Read the model definition and answer for the solid it produces. Units are mm, in the model's axes. A direction names the side the tool comes from. Coordinates: 2 decimals unless noted, no trailing zeros. Loops run counter-clockwise (first coordinate to the right, second up) from the corner with the lowest first, then second, coordinate; pieces in that order, holes last. Notation, with made-up numbers: M 26,62.5 L 39,62.5 A19 cw 39,97.5 Z; hole C 18.25,44.5 d10. An arc over 180 degrees is marked long. Put each result on its own line as item: value.
from build123d import *

# Parameters (mm, degrees)
F1_DEPTH = 38.1
F5_DEPTH = 38.1
F6_DEPTH = 38.1
F7_W     = 25.4
F7_H     = 7.62
F8_DEPTH = 38.1


with BuildPart() as f1:
    # F0 (on Front) → F1 (new body)
    with BuildSketch(Plane.XZ):
        Polygon((6.35, 38.1), (0, 0), (6.35, 0), (11.43, 22.225), (16.51, 9.525), (21.59, 9.525), (26.67, 22.225), (31.75, 0), (38.1, 0), (31.75, 38.1), (25.4, 38.1), (19.05, 22.225), (12.7, 38.1), align=None)
        Polygon((0, 38.1), (0, 0), (6.35, 38.1), align=None)
        Polygon((11.43, 22.225), (6.35, 0), (31.75, 0), (26.67, 22.225), (21.59, 9.525), (16.51, 9.525), align=None)
        Polygon((25.4, 38.1), (12.7, 38.1), (19.05, 22.225), align=None)
        Polygon((31.75, 38.1), (38.1, 0), (38.1, 38.1), align=None)
    extrude(amount=F1_DEPTH)

    # F4 (on offset) → F5 (cut)
    with BuildSketch(Plane.YZ.offset(38.1)):
        Polygon((-31.75, 0), (-38.1, 38.1), (-38.1, 0), align=None)
        Polygon((-11.43, 17.450867), (-6.35, 38.1), (-31.75, 38.1), (-26.67, 17.417177), (-21.59, 28.575), (-16.51, 28.575), align=None)
        Polygon((-25.4, 0), (-12.7, 0), (-19.05, 15.875), align=None)
        Polygon((-6.35, 0), (0, 0), (0, 38.1), align=None)
    extrude(amount=-F5_DEPTH, mode=Mode.SUBTRACT)

    # F0 (on Front) → F6 (cut)
    with BuildSketch(Plane.XZ):
        Polygon((31.75, 38.1), (38.1, 0), (38.1, 38.1), align=None)
        Polygon((25.4, 38.1), (12.7, 38.1), (19.05, 22.225), align=None)
        Polygon((0, 38.1), (0, 0), (6.35, 38.1), align=None)
        Polygon((11.43, 22.225), (6.35, 0), (31.75, 0), (26.67, 22.225), (21.59, 9.525), (16.51, 9.525), align=None)
    extrude(amount=F6_DEPTH, mode=Mode.SUBTRACT)

    # F7 (on offset) → F8 (cut)
    with BuildSketch(Plane.XY.offset(38.1)):
        with Locations((12.7, -26.67)):
            Rectangle(F7_W, F7_H)
        with Locations((25.4, -11.43)):
            Rectangle(F7_W, F7_H)
    extrude(amount=-F8_DEPTH, mode=Mode.SUBTRACT)


solid = f1.part
1) Find section B-B, the plane z = 30. Write down the section's boundary in (x, y), plus the area to 3 significant figures.
Answer list:
outline: M 5,-36.75 L 15.94,-36.75 L 15.94,-30.48 L 5,-30.48 Z; M 5,-8.34 L 12.7,-8.34 L 12.7,-7.62 L 15.94,-7.62 L 15.94,-1.35 L 5,-1.35 Z; M 22.16,-36.75 L 33.1,-36.75 L 33.1,-29.76 L 25.4,-29.76 L 25.4,-30.48 L 22.16,-30.48 Z; M 22.16,-7.62 L 33.1,-7.62 L 33.1,-1.35 L 22.16,-1.35 Z
area: 285 mm^2
2) Find section A-A, the plane x = 36. Write down the section's boundary in (y, z), plus the area to 3 significant figures.
Answer list:
outline: M -33.85,12.6 L -31.75,0 L -25.4,0 L -20.36,12.6 Z; M -17.74,12.6 L -15.24,6.35 L -15.24,12.6 Z; M -7.62,0 L -6.35,0 L -4.25,12.6 L -7.62,12.6 Z
area: 162 mm^2
3) Determine the mould class of faces 4 (the flat face through (35, -7, 0)), 5 (the flat face through (12.7, -14, 21)), 6 (the flat face through (28, -19, 28.575)) for opening direction Y: released by +Y, released by -Y, zero draft, split by the parting line, or undercut.
Answer list:
face 4: zero draft
face 5: undercut
face 6: undercut
4) Given pin 1 Ø2.5 at (x, y) = (8.5, -18.5) entering from +Z (3 decimals); pin 2 Ø1.5 at (y, z) = (-14, 8) entering from +X; pin 3 Ø6 at (x, z) = (14.5, 13) entering from -Y; pin 4 Ø1 at (y, z) = (-28.5, 29.5) entering from -X, each flat-ended and moving along its own axis, determine where each tip first touches the part or whether it passes through.
Answer list:
pin 1: stops at z = 28.575
pin 2: stops at x = 8.35
pin 3: stops at y = -34.42
pin 4: passes through
5) Straight lines are drawn through the part: line 1 (Y direction, x = 8.5, z = 22.5); line 2 (Y direction, x = 5, z = 11.5); line 3 (Y direction, x = 21, z = 11). For each, find the intervals that lie inside material, in ascending order. Write a range as [from, to].
Answer list:
line 1: y = [-35.5, -30.48], [-22.86, -13.74], [-10.19, -2.6]
line 2: y = [-33.67, -30.48], [-22.86, -20.8], [-17.3, -4.43]
line 3: y = [-33.58, -30.48], [-22.86, -21], [-17.1, -15.24], [-7.62, -4.52]
6) Which of the six approach directions +Z, -Z, +X, -X, +Y, -Y give full straight-line access (tool end or side, diameter ignored) to faces 1 (the flat face through (6, -21, 11)), 2 (the flat face through (19, -6, 9.525)), 3 (the flat face through (15.83, -33.39, 30.27))?
Answer list:
face 1: -Z, +X, -X
face 2: -Z, +Y, -Y
face 3: +Z, +Y, -Y
7) Find section C-C, the plane y = -7. Write down the section's boundary in (x, z) (3 decimals), plus the area to 3 significant figures.
Answer list:
outline: M 0,0 L 6.35,0 L 11.43,22.225 L 16.51,9.525 L 21.59,9.525 L 26.67,22.225 L 31.75,0 L 38.1,0 L 32.19,35.458 L 24.343,35.458 L 19.05,22.225 L 13.757,35.458 L 5.91,35.458 Z
area: 749 mm^2
